```python
from build123d import *

# Parameters (mm, degrees)
F0_R     = 1.78928
F0_R_2   = 11.303
F1_DEPTH = 6.35
F2_R     = 1.27


with BuildPart() as f1:
    # F0 (on Top) → F1 (new body)
    with BuildSketch(Plane.XY):
        with BuildLine():
            ThreePointArc((12.077109, 10.303352), (9.095838, 15.699831), (8.080235, 21.780827))
            ThreePointArc((8.080235, 21.780827), (0, 17.78), (-8.080235, 21.780827))
            ThreePointArc((-8.080235, 21.780827), (-9.074817, 15.723861), (-12.038361, 10.348599))
            ThreePointArc((-12.038361, 10.348599), (0.029785, 15.874972), (12.077109, 10.303352))
        make_face()
        with BuildLine():
            ThreePointArc((10.16, 27.94), (7.184205, 35.124205), (0, 38.1))
            ThreePointArc((0, 38.1), (-0.87291, 38.039306), (-1.743288, 37.949323))
            ThreePointArc((-1.743288, 37.949323), (-9.459411, 31.647444), (-8.080235, 21.780827))
            ThreePointArc((-8.080235, 21.780827), (0, 17.78), (8.080235, 21.780827))
            ThreePointArc((8.080235, 21.780827), (9.626027, 24.689583), (10.16, 27.94))
        make_face()
        Polygon((-7.112, 32.046115), (0, 36.15223), (7.112, 32.046115), (7.112, 23.833885), (0, 19.72777), (-7.112, 23.833885), align=None, mode=Mode.SUBTRACT)
        with BuildLine():
            ThreePointArc((-8.080235, 21.780827), (-9.459411, 31.647444), (-1.743288, 37.949323))
            ThreePointArc((-1.743288, 37.949323), (-12.66546, 34.030722), (-20.801573, 25.757091))
            ThreePointArc((-20.801573, 25.757091), (-13.884792, 25.548137), (-8.080235, 21.780827))
        make_face()
        with Locations((-12.453423, 30.944496)):
            Circle(F0_R, mode=Mode.SUBTRACT)
        with BuildLine():
            ThreePointArc((2.348846, -15.700272), (2.616295, -15.653525), (2.88441, -15.610759))
            ThreePointArc((2.88441, -15.610759), (12.202574, -10.154448), (15.875, 0))
            ThreePointArc((15.875, 0), (15.649988, 2.663364), (14.98133, 5.251227))
            ThreePointArc((14.98133, 5.251227), (14.873941, 5.532726), (14.771257, 5.815976))
            ThreePointArc((14.771257, 5.815976), (13.748153, 7.9375), (12.422412, 9.884296))
            ThreePointArc((12.422412, 9.884296), (12.248203, 10.092541), (12.077109, 10.303352))
            ThreePointArc((12.077109, 10.303352), (0.029785, 15.874972), (-12.038361, 10.348599))
            ThreePointArc((-12.038361, 10.348599), (-12.228452, 10.114848), (-12.422412, 9.884296))
            ThreePointArc((-12.422412, 9.884296), (-13.748153, 7.9375), (-14.771257, 5.815976))
            ThreePointArc((-14.771257, 5.815976), (-14.864498, 5.560985), (-14.961519, 5.307407))
            ThreePointArc((-14.961519, 5.307407), (-13.763022, -7.911691), (-2.942969, -15.599826))
            ThreePointArc((-2.942969, -15.599826), (-2.645489, -15.647574), (-2.348846, -15.700272))
            ThreePointArc((-2.348846, -15.700272), (0, -15.875), (2.348846, -15.700272))
        make_face()
        Circle(F0_R_2, mode=Mode.SUBTRACT)
        with BuildLine():
            ThreePointArc((-22.902867, -3.892725), (-32.653508, -8.33894), (-32.995568, -19.05))
            ThreePointArc((-32.995568, -19.05), (-32.50655, -19.775615), (-31.993434, -20.484393))
            ThreePointArc((-31.993434, -20.484393), (-22.677785, -24.015812), (-14.822632, -17.888102))
            ThreePointArc((-14.822632, -17.888102), (-14.235158, -15.96807), (-14.03675, -13.97))
            ThreePointArc((-14.03675, -13.97), (-16.568793, -7.258825), (-22.902867, -3.892725))
        make_face()
        Polygon((-17.08475, -9.863885), (-17.08475, -18.076115), (-24.19675, -22.18223), (-31.30875, -18.076115), (-31.30875, -9.863885), (-24.19675, -5.75777), align=None, mode=Mode.SUBTRACT)
        with BuildLine():
            ThreePointArc((-14.961519, 5.307407), (-18.144371, 0.027311), (-22.902867, -3.892725))
            ThreePointArc((-22.902867, -3.892725), (-16.568793, -7.258825), (-14.03675, -13.97))
            ThreePointArc((-14.03675, -13.97), (-14.235158, -15.96807), (-14.822632, -17.888102))
            ThreePointArc((-14.822632, -17.888102), (-9.079854, -15.720953), (-2.942969, -15.599826))
            ThreePointArc((-2.942969, -15.599826), (-13.763022, -7.911691), (-14.961519, 5.307407))
        make_face()
        with BuildLine():
            ThreePointArc((-14.822632, -17.888102), (-22.677785, -24.015812), (-31.993434, -20.484393))
            ThreePointArc((-31.993434, -20.484393), (-23.13874, -27.983971), (-11.905509, -30.893236))
            ThreePointArc((-11.905509, -30.893236), (-15.182939, -24.798651), (-14.822632, -17.888102))
        make_face()
        with Locations((-20.572009, -26.257229)):
            Circle(F0_R, mode=Mode.SUBTRACT)
        with BuildLine():
            ThreePointArc((2.88441, -15.610759), (9.048534, -15.727142), (14.822632, -17.888102))
            ThreePointArc((14.822632, -17.888102), (15.397932, -8.89), (22.902867, -3.892725))
            ThreePointArc((22.902867, -3.892725), (18.154672, -0.002908), (14.98133, 5.251227))
            ThreePointArc((14.98133, 5.251227), (15.649988, 2.663364), (15.875, 0))
            ThreePointArc((15.875, 0), (12.202574, -10.154448), (2.88441, -15.610759))
        make_face()
        with BuildLine():
            ThreePointArc((14.822632, -17.888102), (23.548488, -24.109298), (32.995568, -19.05))
            ThreePointArc((32.995568, -19.05), (33.37946, -18.263691), (33.736722, -17.46493))
            ThreePointArc((33.736722, -17.46493), (34.200542, -15.744752), (34.35675, -13.97))
            ThreePointArc((34.35675, -13.97), (30.907925, -6.342043), (22.902867, -3.892725))
            ThreePointArc((22.902867, -3.892725), (15.397932, -8.89), (14.822632, -17.888102))
        make_face()
        Polygon((17.08475, -9.863885), (24.19675, -5.75777), (31.30875, -9.863885), (31.30875, -18.076115), (24.19675, -22.18223), (17.08475, -18.076115), align=None, mode=Mode.SUBTRACT)
        with BuildLine():
            ThreePointArc((34.35675, -13.97), (34.200542, -15.744752), (33.736722, -17.46493))
            ThreePointArc((33.736722, -17.46493), (35.8042, -6.046751), (32.707082, 5.136145))
            ThreePointArc((32.707082, 5.136145), (29.067732, -0.749485), (22.902867, -3.892725))
            ThreePointArc((22.902867, -3.892725), (30.907925, -6.342043), (34.35675, -13.97))
        make_face()
        with Locations((33.025431, -4.687268)):
            Circle(F0_R, mode=Mode.SUBTRACT)
    extrude(amount=F1_DEPTH)

    # F2
    f2_edges = [f1.edges().sort_by_distance(p)[0] for p in [
        (-20.801573, 25.757091, 3.175),
        (-11.905509, -30.893236, 3.175),
        (32.707082, 5.136145, 3.175),
    ]]
    fillet(f2_edges, radius=F2_R)


solid = f1.part
```
Build history of the part. All positions in model axes, mm. A direction names the side the tool comes from. Give positions to 0.01 mm unless a question says otherwise; leave off trailing zeros. Loops run counter-clockwise (first coordinate to the right, second up) from the corner with the lowest first, then second, coordinate; pieces in that order, holes last. Notation, with made-up numbers: (0.5, 32.5) -> (32.5, 32.5) arc R17 ccw to (32.5, 58.5) -> close; hole circle Ø9 at (72.5, -35). An arc over 180 degrees is marked (long way). One line per question, with ' | ' between items. Start each with the question number.
1) Cut at A-A (x = 30). Give the cut face in (y, z).
2) Cut at B-B (y = 0). Give the cut face in (x, z), plus the area to 3 significant figures.
3) 3-axis set-ups, long thin cutter, end or side, ignore diameter. For faces 1 (the cylindrical face through (-0.033, -15.875, 3.131)), 2 (the flat face through (-3.506, 21.752, 3.131)), 3 (the cylindrical face through (9.125, 15.618, 3.131)): which of +Z, -Z, +X, -X, +Y, -Y reach the whole face in a straight line?
4) Two-plate mould, pull along X, no slides. Class faces 4 (the flat face through (-17.085, -14, 3)), 5 (the cylindrical face through (35.828, -7.669, 3.131)), 6 (the cylindrical face through (-9.047, 15.806, 3.131)): released by +X, released by -X, zero draft, split by the parting line, or undercut.
5) Pin check, flat tips, straight feed: pin 1 (1.9 mm diameter, centred on y = 26, z = 2.5, fed in from -X); pin 2 (3 mm diameter, centred on y = -14.5, z = 2, fed in from +X); pin 3 (3 mm diameter, centred on y = -13.5, z = 1.5, fed in from +X). Stop position of each tip, or through.
6) Cut at D-D (z = 1.75). Count the separate pieces of the cut face and the enclosed holes in it, plus the area to 3 significant figures.
7) Cut at C-C (x = -5.5). Give the cut face in (y, z).
8) Probe L1, parallel to Y at x = 5, z = 0.5; L2, parallel to Y at x = 3.5, z = 2.5; L3, parallel to X at y = -17, z = 5.75. List the from-to ranges inside material, lowest first.
Return value:
1) outline: (-22.31, 0) -> (-18.83, 0) -> (-18.83, 6.35) -> (-22.31, 6.35) -> close; (-9.11, 0) -> (0.2, 0) -> (0.2, 6.35) -> (-9.11, 6.35) -> close
2) outline: (-18.17, 0) -> (-11.3, 0) -> (-11.3, 6.35) -> (-18.17, 6.35) -> close; (11.3, 0) -> (18.15, 0) -> (18.15, 6.35) -> (11.3, 6.35) -> close; (29.82, 0) -> (34.81, 0) -> (34.81, 6.35) -> (29.82, 6.35) -> close | area: 119 mm^2
3) face 1: +Z, -Z, -Y | face 2: +Z, -Z | face 3: +Z, -Z, +X
4) face 4: undercut | face 5: released by +X | face 6: released by -X
5) pin 1: x = -19.3 | pin 2: x = 35.18 | pin 3: x = 35.39
6) separate pieces: 1 | enclosed holes: 7 | area: 1,260 mm^2
7) outline: (-15.4, 0) -> (-9.87, 0) -> (-9.87, 6.35) -> (-15.4, 6.35) -> close; (9.87, 0) -> (22.9, 0) -> (22.9, 6.35) -> (9.87, 6.35) -> close; (32.98, 0) -> (37.21, 0) -> (37.21, 6.35) -> (32.98, 6.35) -> close
8) L1: -15.41 to -10.14, 10.14 to 22.61, 33.27 to 36.78 | L2: -15.53 to -10.75, 10.75 to 21.75, 34.13 to 37.48 | L3: -33.89 to -31.31, -17.08 to -13.11, 13.09 to 17.08, 31.31 to 33.93
